Autodesk Inventor part; units mm, degrees
ref_plane "YZ Plane" through (0, 0, 0) normal (1, 0, 0) x (0, 1, 0)
ref_plane "XZ Plane" through (0, 0, 0) normal (0, 1, 0) x (-1, 0, 0)
ref_plane "XY Plane" through (0, 0, 0) normal (0, 0, 1) x (1, 0, 0)
sketch "Skizze2" plane through (0, 0, 0) normal (0, 0, 1) x (1, 0, 0)
  line L0 (0, 18) -> (35, 18)
  line L1 (35, 18) -> (35, 0)
  line L2 (35, 0) -> (0, 0)
  line L3 (0, 0) -> (0, 18)
  dimension "d12" = 18
  dimension "d13" = 35
extrude "Grobblech2" add sketch "Skizze2" along normal blind 0.5
sketch "Skizze3" plane through (0, 17.5, 0) normal (0, 1, 0) x (-1, 0, 0)
  line L0 (-35, 0) -> (0, 0)
  line L1 (0, 0) -> (0, 18)
  line L2 (0, 18) -> (-35, 18)
  line L3 (-35, 18) -> (-35, 0)
edge flange "Lasche1" height 18 angle 90 thickness 0.5 bend radius 0.5 thickness toward (0, 1, 0) relief tear relief width 0.5 relief depth 0.25 edges at (17.5, 18, 0.5) wall of the first edge with corners at (35, 17.5, 0) (0, 17.5, 0) (0, 17.5, 18) (35, 17.5, 18)
bend "Biegung1"
corner "Ecke1"
sketch "Skizze4" plane through (35, 0.5, 0) normal (0, -1, 0) x (1, 0, 0)
  line L0 (-35, 0) -> (0, 0)
  line L1 (0, 0) -> (0, 18)
  line L2 (0, 18) -> (-35, 18)
  line L3 (-35, 18) -> (-35, 0)
edge flange "Lasche2" height 18 angle 90 thickness 0.5 bend radius 0.5 thickness toward (0, -1, 0) relief tear relief width 0.5 relief depth 0.25 edges at (17.5, 0, 0.5) wall of the first edge with corners at (0, 0.5, 0) (35, 0.5, 0) (35, 0.5, 18) (0, 0.5, 18)
bend "Biegung2"
corner "Ecke2"
sketch "Skizze5" plane through (35, 17.5, 17.5) normal (0, 0, 1) x (1, 0, 0)
  line L0 (-35, 0) -> (0, 0)
  line L1 (0, 0) -> (0, 15.5)
  line L2 (0, 15.5) -> (-35, 15.5)
  line L3 (-35, 15.5) -> (-35, 0)
edge flange "Lasche3" height 15.5 angle 90 thickness 0.5 bend radius 0.5 thickness toward (0, 0, 1) relief tear relief width 0.5 relief depth 0.25 edges at (17.5, 18, 18) wall of the first edge with corners at (0, 17.5, 17.5) (35, 17.5, 17.5) (35, 33, 17.5) (0, 33, 17.5)
bend "Biegung3"
corner "Ecke3"
sketch "Skizze6" plane through (0, 0.5, 17.5) normal (0, 0, 1) x (1, 0, 0)
  line L0 (35, 0) -> (0, 0)
  line L1 (0, 0) -> (0, -15.5)
  line L2 (0, -15.5) -> (35, -15.5)
  line L3 (35, -15.5) -> (35, 0)
edge flange "Lasche4" height 15.5 angle 90 thickness 0.5 bend radius 0.5 thickness toward (0, 0, 1) relief tear relief width 0.5 relief depth 0.25 edges at (17.5, 0, 18) wall of the first edge with corners at (35, 0.5, 17.5) (0, 0.5, 17.5) (0, -15, 17.5) (35, -15, 17.5)
bend "Biegung4"
corner "Ecke4"
sketch "Skizze7" plane through (0, 0, 1) normal (0, -1, 0) x (1, 0, 0)
  line L0 (35, -1) -> (21, -1)
  line L1 (21, -1) -> (21, 3)
  line L2 (21, 3) -> (35, 3)
  line L3 (35, 3) -> (35, -1)
  line L4 (35, -1) -> (0, -1)
  dimension "d55" = 4
  dimension "d56" = 14
extrude "Ausschneiden1" cut sketch "Skizze7" against normal up to surface (18 mm away)
sketch "Skizze8" plane through (0, 0, 0) normal (0, 0, -1) x (-1, 0, 0)
  line L0 (-21, 17) -> (-21, 1)
  line L1 (-21, 1) -> (0, 1)
  line L2 (0, 17) -> (0, 1)
  line L3 (0, 17) -> (-21, 17)
  line L4 (0, 9) -> (-30.5159, 9) construction
  line L5 (-35, -15) -> (0, -15)
  line L6 (-17.5, -15) -> (-17.5, 33) construction
  line L7 (0, 33) -> (-35, 33)
  point P0 (0, 0)
  point P1 (-30, 28)
  point P2 (-5, 28)
  point P3 (-30, -10)
  point P4 (-5, -10)
  dimension "d59" = 25
  dimension "d60" = 38
  dimension "d61" = 25
  dimension "d62" = 38
hole "Bohrung1" at (30, 28, 0) at (5, 28, 0) at (30, -10, 0) at (5, -10, 0) direction (0, 0, 1) diameter 4.5 depth 18
sketch "Skizze9" plane through (0, 0, 0) normal (0, 0, -1) x (-1, 0, 0)
  line L0 (0, 17) -> (0, 1)
  point P0 (0, 0)
  point P1 (-8, 8.1851)
  point P2 (-16, 8.1851)
  dimension "d70" = 8
  dimension "d71" = 8
hole "Bohrung2" at (8, 8.1851, 0) at (16, 8.1851, 0) direction (0, 0, 1) diameter 3 end through all
equation "\"d57\" = Stärke"
equation "\"d68\" = Stärke"
equation "\"d14\" = Stärke"
equation "\"d15\" = BreiteBiegungsfreistellung"
equation "\"d16\" = TiefeBiegungsfreistellung"
equation "\"d17\" = MinimalRest"
equation "\"d18\" = Übergangsradius"
equation "\"d21\" = Biegeradius"
equation "\"d22\" = GrößeEckenfreistellung"
equation "\"d23\" = Abstandsgröße"
equation "\"d24\" = JacobiRadiusGröße"
equation "\"d25\" = BreiteBiegungsfreistellung"
equation "\"d26\" = TiefeBiegungsfreistellung"
equation "\"d27\" = MinimalRest"
equation "\"d28\" = Übergangsradius"
equation "\"d31\" = Biegeradius"
equation "\"d32\" = GrößeEckenfreistellung"
equation "\"d33\" = Abstandsgröße"
equation "\"d34\" = JacobiRadiusGröße"
equation "\"d35\" = BreiteBiegungsfreistellung"
equation "\"d36\" = TiefeBiegungsfreistellung"
equation "\"d37\" = MinimalRest"
equation "\"d38\" = Übergangsradius"
equation "\"d41\" = Biegeradius"
equation "\"d42\" = GrößeEckenfreistellung"
equation "\"d43\" = Abstandsgröße"
equation "\"d44\" = JacobiRadiusGröße"
equation "\"d45\" = BreiteBiegungsfreistellung"
equation "\"d46\" = TiefeBiegungsfreistellung"
equation "\"d47\" = MinimalRest"
equation "\"d48\" = Übergangsradius"
equation "\"d51\" = Biegeradius"
equation "\"d52\" = GrößeEckenfreistellung"
equation "\"d53\" = Abstandsgröße"
equation "\"d54\" = JacobiRadiusGröße"
equation "\"Biegeradius\" = Stärke"
equation "\"BreiteBiegungsfreistellung\" = Stärke"
equation "\"TiefeBiegungsfreistellung\" = 0.5 * Stärke"
equation "\"GrößeEckenfreistellung\" = 4 * Stärke"
equation "\"MinimalRest\" = 2 * Stärke"
equation "\"Übergangsradius\" = Biegeradius"
equation "\"JacobiRadiusGröße\" = Biegeradius"
equation "\"Abstandsgröße\" = Stärke"
properties part number "Bügelbefestigung" material "Stahl, galvanisiert"
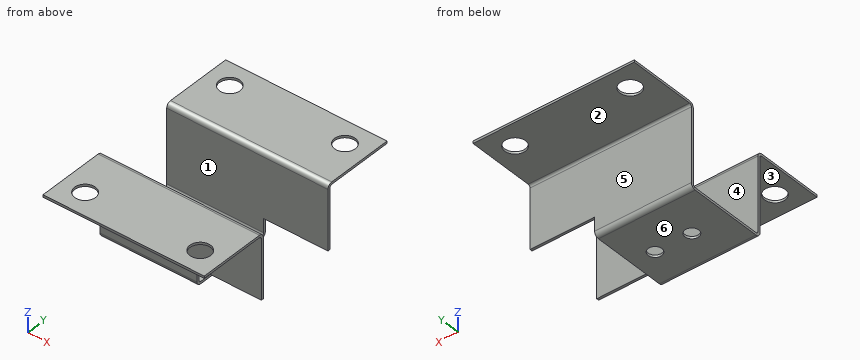
Verification items for the finished model (mm, model axes). Face numbers are marked on the shaded views. A direction names the side the tool comes from. Round coordinates to 2 decimals unless told otherwise and drop trailing zeros. Write each loop counter-clockwise with the first axis right and the second up, starting at its lowest first coordinate (ties: lowest second). Pieces come first, ordered by that corner, then holes.
(1) Section check A-A (z = 10.5). Enter the section's corners in (x, y).
Returned:
outline: (0, 0) - (35, 0) - (35, 0.5) - (0, 0.5) - close; (0, 17.5) - (35, 17.5) - (35, 18) - (0, 18) - close
(2) Material ranges on line 1 (X direction, y = -10, z = 17.65); line 2 (Y direction, x = 14, z = 12.75); line 3 (Y direction, x = 5, z = 17.9), recorded low to high.
Returned:
line 1: x = 0 to 2.75, 7.25 to 27.75, 32.25 to 35
line 2: y = 0 to 0.5, 17.5 to 18
line 3: y = -15 to -12.25, -7.75 to -0.06, 18.06 to 25.75, 30.25 to 33
(3) Section check D-D (y = -10). Enter the section's corners in (x, z), plus the area to 3 significant figures.
Returned:
outline: (0, 17.5) - (2.75, 17.5) - (2.75, 18) - (0, 18) - close; (7.25, 17.5) - (27.75, 17.5) - (27.75, 18) - (7.25, 18) - close; (32.25, 17.5) - (35, 17.5) - (35, 18) - (32.25, 18) - close
area: 13.0 mm2
(4) Mould release check, pull along Y, two halves, no side actions. Record for the marked faces 4, 5 and 6: pulls with the +Y half, pulls with the -Y half, needs draft (parallel to the pull), parting line crosses it, or undercut.
Returned:
face 4: undercut
face 5: pulls with the +Y half
face 6: needs draft
(5) Depth check by flat-ended pin: pin 1 Ø8 at (x, z) = (23.5, 4) entering from -Y; pin 2 Ø3.5 at (x, y) = (16, 8.19) entering from +Z; pin 3 Ø16 at (x, y) = (23, -11) entering from -Z; pin 4 Ø1 at (y, z) = (19.5, 5) entering from -X. Enter the tip coordinate at first touch or a pass-through.
Returned:
pin 1: stops at y = 0
pin 2: stops at z = 0.5
pin 3: stops at z = 17.5
pin 4: passes through
(6) Section check C-C (x = 30). Enter the section's corners in (y, z).
Returned:
outline: (-15, 17.5) - (-12.25, 17.5) - (-12.25, 18) - (-15, 18) - close; (-7.75, 17.5) - (-0.5, 17.5) arc R0.5 cw to (0, 17) - (0, 4) - (0.5, 4) - (0.5, 17) arc R1 ccw to (-0.5, 18) - (-7.75, 18) - close; (17.5, 4) - (18, 4) - (18, 17) arc R0.5 cw to (18.5, 17.5) - (25.75, 17.5) - (25.75, 18) - (18.5, 18) arc R1 ccw to (17.5, 17) - close; (30.25, 17.5) - (33, 17.5) - (33, 18) - (30.25, 18) - close
(7) Access from +Z, -Z, +X, -X, +Y, -Y to the whole of each face (thin tool, end or side, straight path). Record for the marked faces 1, 2 and 3.
Returned:
face 1: +Z, +X, -X
face 2: -Z, +X, -X, +Y
face 3: -Z, +X, -X, -Y
(8) Section check B-B (x = 22). Enter the section's corners in (y, z), plus the area to 3 significant figures.
Returned:
outline: (-15, 17.5) - (-0.5, 17.5) arc R0.5 cw to (0, 17) - (0, 4) - (0.5, 4) - (0.5, 17) arc R1 ccw to (-0.5, 18) - (-15, 18) - close; (17.5, 4) - (18, 4) - (18, 17) arc R0.5 cw to (18.5, 17.5) - (33, 17.5) - (33, 18) - (18.5, 18) arc R1 ccw to (17.5, 17) - close
area: 28.7 mm2
